The drawing under review shows one solid part. Ordinate dimensions are in mm from its lowest x, y, z. A direction names the side the tool comes from. Give positions to 0.01 mm unless a question says otherwise; leave off trailing zeros. Write each loop counter-clockwise with the first axis right and the second up, starting at its lowest first coordinate (ties: lowest second). Pieces come first, ordered by that corner, then holes.
Q1. For line 1 (Z direction, x = 4.75, y = 8.75); line 2 (Y direction, x = 5.75, z = 1.5) (1 decimal); line 3 (Z direction, x = 3.75, y = 3), list the stretches that pass through material, from the lowest coordinate up.
Q2. Insertion check: P1, Ø0.7, axis at y = 5.5, z = 1.5, coming from the -X side; P2, Ø0.8, axis at x = 5, y = 5, coming from the -Z side; P3, Ø1, axis at x = 6, z = 9.5, coming from the +Y side. Each pin has a flat end and moves straight along its axis. Give the tip position at first contact, or say it passes through.
Q3. Machinability: for the marked faces 4 and 5, which of the approach directions +Z, -Z, +X, -X, +Y, -Y give a long, thin tool a straight path to every point of the face, cutting with its end or side? Answer none if there is none.
Q4. We need section A-A (y = 5). Write out the cut boundary in (x, z), then the cut area to 3 significant figures.
Q5. We need section C-C (x = 1). Write out the cut boundary in (y, z), then the cut area to 3 significant figures.
Q6. We need section B-B (z = 9.75). Write out the cut boundary in (x, y), then the cut area to 3 significant figures.
Q7. Mouldability with a two-part tool opening along Y and no side actions: class the marked faces 1, 2 and 3 as released by +Y, released by -Y, zero draft, split by the parting line, or undercut.
Q8. We need section D-D (y = 7.5). Write out the cut boundary in (x, z).
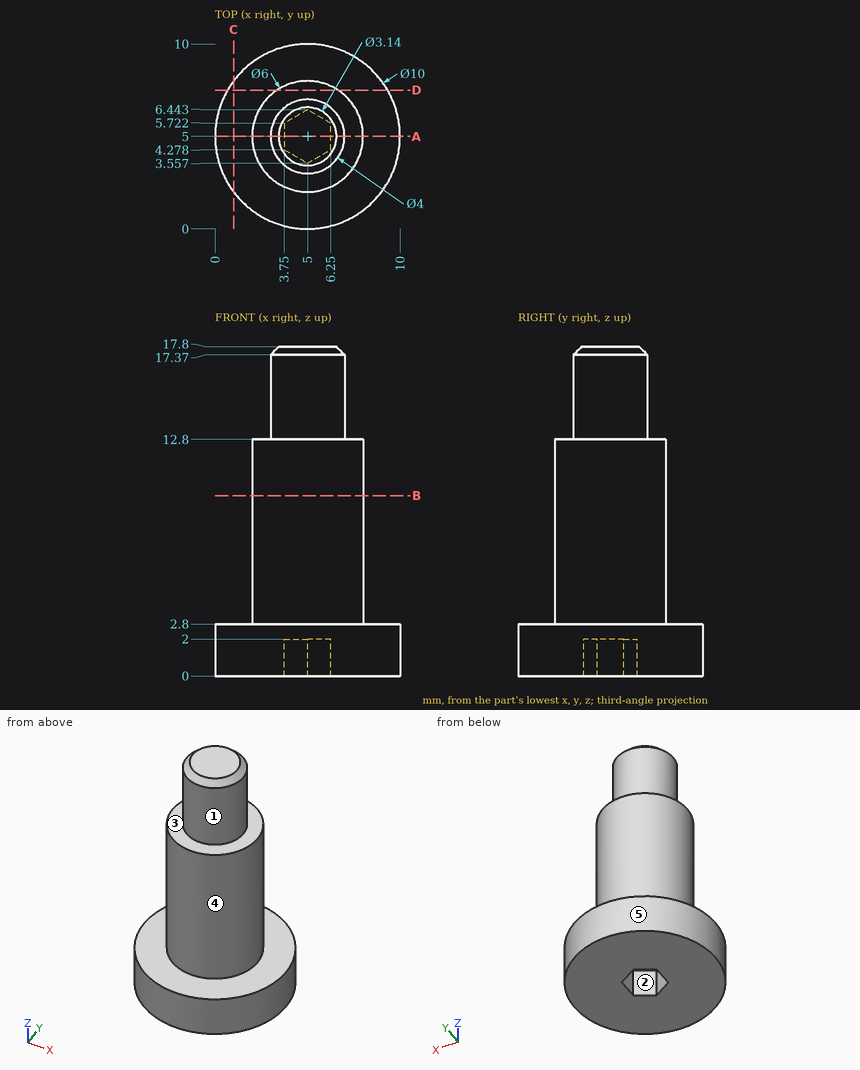
Computed:
1. line 1: z = 0 to 2.8
1. line 2: y = 0.1 to 4, 6 to 9.9
1. line 3: z = 0 to 12.8
2. P1: stops at x = 0
2. P2: stops at z = 2
2. P3: stops at y = 7.96
3. face 4: +Z
3. face 5: +Z, -Z
4. outline: (0, 0) - (3.75, 0) - (3.75, 2) - (6.25, 2) - (6.25, 0) - (10, 0) - (10, 2.8) - (8, 2.8) - (8, 12.8) - (7, 12.8) - (7, 17.37) - (6.57, 17.8) - (3.43, 17.8) - (3, 17.37) - (3, 12.8) - (2, 12.8) - (2, 2.8) - (0, 2.8) - close
4. area: 103 mm2
5. outline: (2, 0) - (8, 0) - (8, 2.8) - (2, 2.8) - close
5. area: 16.8 mm2
6. outline: circle Ø6 at (5, 5)
6. area: 28.3 mm2
7. face 1: split by the parting line
7. face 2: undercut
7. face 3: zero draft
8. outline: (0.67, 0) - (9.33, 0) - (9.33, 2.8) - (6.66, 2.8) - (6.66, 12.8) - (3.34, 12.8) - (3.34, 2.8) - (0.67, 2.8) - close
